Could you check a few things on this model? Use its own coordinates, in mm. A direction names the side the tool comes from. Give positions to 0.01 mm unless a question says otherwise; leave off trailing zeros. Loops run counter-clockwise (first coordinate to the right, second up) from the corner with the lowest first, then second, coordinate; pieces in that order, holes last. Notation, with made-up numbers: M 74,78 L 93,78 A16 ccw 93,109 Z; hole C 45,24.25 d2. An arc over 180 degrees is marked long. Use a Markdown table: item, result. Add a question column.
1) We'd pull the mould along X, two halves only. Please class faces 5 (the cylindrical face through (39.536, 1.014, -3.825)), 6 (the cylindrical face through (39.67, 1.01, -40.01)), 7 (the flat face through (22, 1, -44)), 8 (the flat face through (16, 5, -7)): +X half, -X half, draft (parallel to the pull), parting line (faces both ways), or undercut.
2) Will these pins go through, and if not, where does the flat tip stop? pin 1 Ø1.6 at (x, y) = (32, 1.5) entering from +Z; pin 2 Ø5 at (x, z) = (39, -5) entering from +Y; pin 3 Ø5 at (x, y) = (11, 5) entering from -Z.
3) Which directions (+Z, -Z, +X, -X, +Y, -Y) give clear straight access to the entire face, cutting with the end or side of a thin tool? Please do faces 1 (the flat face through (9.5, 5, -7)), 2 (the flat face through (13, 5, -13)), 3 (the cylindrical face through (15.248, 5.39, 0.232)), 4 (the flat face through (22, 0, -22)).
4) Suppose I cut it at A-A on x = 3.8. List the corners of the cut face in (y, z) for me.
5) Suppose I cut it at D-D on y = 5.5. List the corners of the cut face in (x, z) for me, and give its area (3 significant figures).
6) Suppose I cut it at C-C on z = -40.7. List the corners of the cut face in (x, y) for me.
7) Suppose I cut it at B-B on z = -3.5. List the corners of the cut face in (x, y) for me.
8) If I drill on line 1 along Y through (x, z) = (24, -16); line 2 along Z through (x, y) = (6, 1); line 3 along Y through (x, z) = (12.5, -7), over which ranges is the centre line in solid material (lowest first)? Write a range as [from, to].
```python
from build123d import *

# Parameters (mm, degrees)
SKETCH1_W           = 44.5
SKETCH1_H           = 44
BOSS_EXTRUDE1_DEPTH = 2
SKETCH2_R           = 1.5
CUT_EXTRUDE1_DEPTH  = 63.611899827
SKETCH3_W           = 6.5
SKETCH3_H           = 12
BOSS_EXTRUDE2_DEPTH = 7
SKETCH4_R           = 2.5
BOSS_EXTRUDE3_DEPTH = 2.5
SKETCH5_R           = 1.920961375
CUT_EXTRUDE2_DEPTH  = 11.5
FILLET1_R           = 1


with BuildPart() as part:
    # Sketch1 → Boss-Extrude1 (new body)
    with BuildSketch(Plane(origin=(0, 0, 0), x_dir=(1, 0, 0), z_dir=(0, 1, 0))):
        with Locations((22.25, 22)):
            Rectangle(SKETCH1_W, SKETCH1_H)
    extrude(amount=BOSS_EXTRUDE1_DEPTH)

    # Sketch2 → Cut-Extrude1 (cut, through all)
    with BuildSketch(Plane(origin=(0, 2, 0), x_dir=(1, 0, 0), z_dir=(0, 1, 0))):
        with Locations(Location((3.8, 40.7, 0), (0, 0, 270))):
            Circle(SKETCH2_R)
        with Locations(Location((3.8, 3.5, 0), (0, 0, 270))):
            Circle(SKETCH2_R)
        with Locations(Location((41, 3.5, 0), (0, 0, 270))):
            Circle(SKETCH2_R)
        with Locations(Location((41, 40.7, 0), (0, 0, 270))):
            Circle(SKETCH2_R)
    extrude(amount=-CUT_EXTRUDE1_DEPTH, mode=Mode.SUBTRACT)

    # Sketch3 → Boss-Extrude2 (add)
    with BuildSketch(Plane(origin=(0, 2, 0), x_dir=(1, 0, 0), z_dir=(0, 1, 0))):
        with Locations((12.75, 7)):
            Rectangle(SKETCH3_W, SKETCH3_H)
    extrude(amount=BOSS_EXTRUDE2_DEPTH)

    # Sketch4 → Boss-Extrude3 (add)
    with BuildSketch(Plane.XY.offset(-1)):
        with Locations(Location((12.75, 5.5, 0), (0, 0, 180))):
            Circle(SKETCH4_R)
    extrude(amount=BOSS_EXTRUDE3_DEPTH)

    # Sketch5 → Cut-Extrude2 (cut)
    with BuildSketch(Plane.XY.offset(1.5)):
        with Locations((12.75, 5.5)):
            Circle(SKETCH5_R)
    extrude(amount=-CUT_EXTRUDE2_DEPTH, mode=Mode.SUBTRACT)

    # Fillet1
    fillet1_edges = [part.edges().sort_by_distance(p)[0] for p in [
        (0, 1, -44),
        (44.5, 1, -44),
        (44.5, 1, 0),
        (0, 1, 0),
    ]]
    fillet(fillet1_edges, radius=FILLET1_R)


solid = part.part
```
Answer block:
| question | item | result |
|---|---|---|
| 1 | face 5 | undercut |
| 1 | face 6 | undercut |
| 1 | face 7 | draft |
| 1 | face 8 | +X half |
| 2 | pin 1 | stops at z = 0 |
| 2 | pin 2 | stops at y = 2 |
| 2 | pin 3 | stops at z = -13 |
| 3 | face 1 | +Z, -Z, -X, +Y |
| 3 | face 2 | -Z, +X, -X, +Y |
| 3 | face 3 | +Z |
| 3 | face 4 | +Z, -Z, +X, -X, -Y |
| 4 | outline | M 0,-44 L 2,-44 L 2,-42.2 L 0,-42.2 Z; M 0,-39.2 L 2,-39.2 L 2,-5 L 0,-5 Z; M 0,-2 L 2,-2 L 2,0 L 0,0 Z |
| 5 | outline | M 9.5,-13 L 16,-13 L 16,-1 L 15.25,-1 L 15.25,1.5 L 14.67,1.5 L 14.67,-10 L 10.83,-10 L 10.83,1.5 L 10.25,1.5 L 10.25,-1 L 9.5,-1 Z |
| 5 | area | 46.3 mm^2 |
| 6 | outline | M 0,0 L 2.3,0 L 2.3,2 L 0,2 Z; M 5.3,0 L 39.5,0 L 39.5,2 L 5.3,2 Z; M 42.5,0 L 44.5,0 L 44.5,2 L 42.5,2 Z |
| 7 | outline | M 0,0 L 2.3,0 L 2.3,2 L 0,2 Z; M 5.3,0 L 39.5,0 L 39.5,2 L 16,2 L 16,9 L 9.5,9 L 9.5,2 L 5.3,2 Z; M 42.5,0 L 44.5,0 L 44.5,2 L 42.5,2 Z; hole C 12.75,5.5 d3.84 |
| 8 | line 1 | y = [0, 2] |
| 8 | line 2 | z = [-44, 0] |
| 8 | line 3 | y = [0, 3.6], [7.4, 9] |
